Can you work these out from the drawing? Everything is in mm from the part's minimum corner. A direction names the side the tool comes from. Coordinates: 2 decimals unless noted, no trailing zeros. Loops run counter-clockwise (first coordinate to the right, second up) from the corner with the lowest first, then second, coordinate; pieces in that order, holes last. Notation, with made-up numbers: M 34.25,64.5 L 75.25,64.5 A31 ccw 75.25,95.5 Z; hole C 80.5,56.5 d10. An arc over 180 degrees is marked long. Use CSV: the item, a comma, the result in double quotes. Start each with the question number.
Q1. For pin 1 Ø6 at (y, z) = (7, 31.5) entering from -X; pin 2 Ø4 at (x, y) = (5.27, 2.5) entering from +Z; pin 3 Ø1.5 at (y, z) = (7.5, 20.5) entering from +X, each with a flat end and sliding along its axis, tell me the tip position at first contact or that it passes through.
Q2. If we section it at A-A (y = 9.5): Please give me the cut outline in (x, z).
Q3. Please list where these lines run through material, in increasing order: probe 1 along Z at (x, y) = (27.5, 6); probe 2 along Z at (x, y) = (23.5, 7.75); probe 3 along X at (y, z) = (6.75, 33). Write a range as [from, to].
Q4. If we section it at D-D (z = 27): Please give me the cut outline in (x, y).
Q5. If we section it at B-B (z = 33): Please give me the cut outline in (x, y), and give its area (3 significant figures).
Q6. Which directions (+Z, -Z, +X, -X, +Y, -Y) give clear straight access to the entire face, cutting with the end or side of a thin tool? Please do the marked faces 1, 2, 3, 4 and 5.
Q7. If we section it at C-C (x = 27.5): Please give me the cut outline in (y, z), and give its area (3 significant figures).
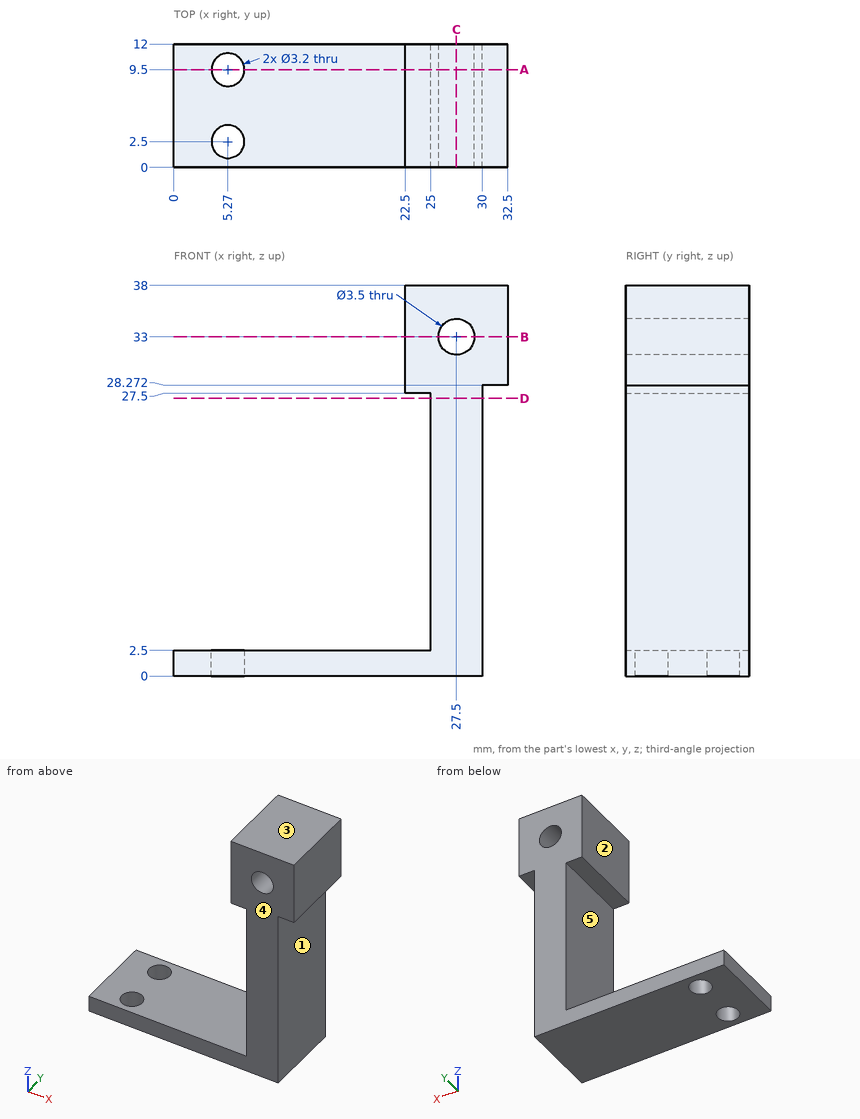
Results below:
1,pin 1,"x = 22.5"
1,pin 2,"z = 2.5"
1,pin 3,"x = 30"
2,outline,"M 0,0 L 3.67,0 L 3.67,2.5 L 0,2.5 Z; M 6.87,0 L 30,0 L 30,28.27 L 32.5,28.27 L 32.5,38 L 22.5,38 L 22.5,27.5 L 25,27.5 L 25,2.5 L 6.87,2.5 Z; hole C 27.5,33 d3.5"
3,probe 1,"[0, 31.25], [34.75, 38]"
3,probe 2,"[0, 2.5], [27.5, 38]"
3,probe 3,"[22.5, 25.75], [29.25, 32.5]"
4,outline,"M 25,0 L 30,0 L 30,12 L 25,12 Z"
5,outline,"M 22.5,0 L 25.75,0 L 25.75,12 L 22.5,12 Z; M 29.25,0 L 32.5,0 L 32.5,12 L 29.25,12 Z"
5,area,"78.0 mm^2"
6,face 1,"-Z, +X, +Y, -Y"
6,face 2,"+Z, -X, +Y, -Y"
6,face 3,"+Z, +X, -X, +Y, -Y"
6,face 4,"+Z, -Z, +X, -X, -Y"
6,face 5,"-X, +Y, -Y"
7,outline,"M 0,0 L 12,0 L 12,31.25 L 0,31.25 Z; M 0,34.75 L 12,34.75 L 12,38 L 0,38 Z"
7,area,"414 mm^2"
